Design review of the part shown in the three views and the two pictorial views. Dimensions are in mm from the part's minimum x, y and z. Round coordinates to 2 decimals unless told otherwise and drop trailing zeros. Order: outer loops, then holes, each group sorted by start corner. A loop starts at its lowest first (then second) coordinate and runs counter-clockwise, first axis right, second up.
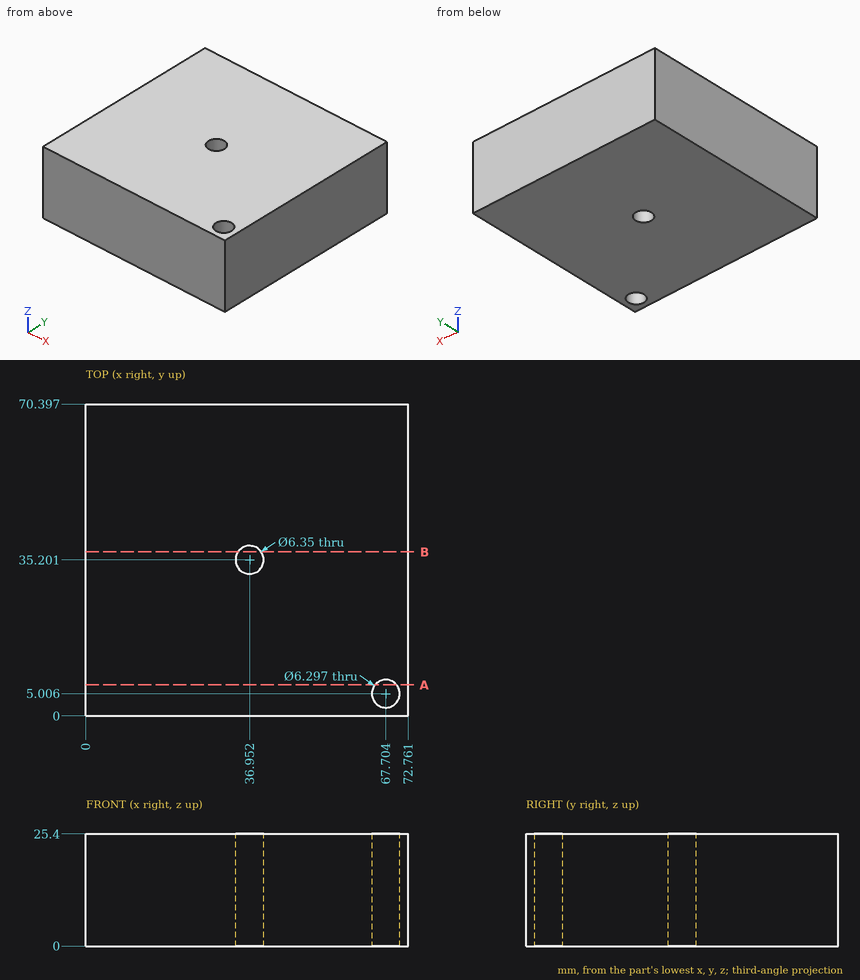
(1) Clearance check with flat-ended pins moving along their axes: P1, Ø5, axis at y = 53, z = 13.5, coming from the -X side; P2, Ø4, axis at x = 67.7, y = 5.01, coming from the +Z side. State where each tip first meets the part, or that it passes through.
(2) Add section A-A on y = 7. Give the boundary of the cut face in (x, z), plus the area to 3 significant figures.
(3) Wall thickness on L1, parallel to X at y = 35.5, z = 6.5; L2, parallel to X at y = 34.5, z = 20 (1 decimal); L3, parallel to Y at x = 37.5, z = 9.25: over which ranges is each line inside the solid? List them lowest first.
(4) Add section B-B on y = 37. Give the boundary of the cut face in (x, z).
Here are the results:
1. P1: stops at x = 0
1. P2: passes through
2. outline: (0, 0) - (65.27, 0) - (65.27, 25.4) - (0, 25.4) - close; (70.14, 0) - (72.76, 0) - (72.76, 25.4) - (70.14, 25.4) - close
2. area: 1,720 mm2
3. L1: x = 0 to 33.79, 40.11 to 72.76
3. L2: x = 0 to 33.9, 40 to 72.8
3. L3: y = 0 to 32.07, 38.33 to 70.4
4. outline: (0, 0) - (34.34, 0) - (34.34, 25.4) - (0, 25.4) - close; (39.57, 0) - (72.76, 0) - (72.76, 25.4) - (39.57, 25.4) - close
